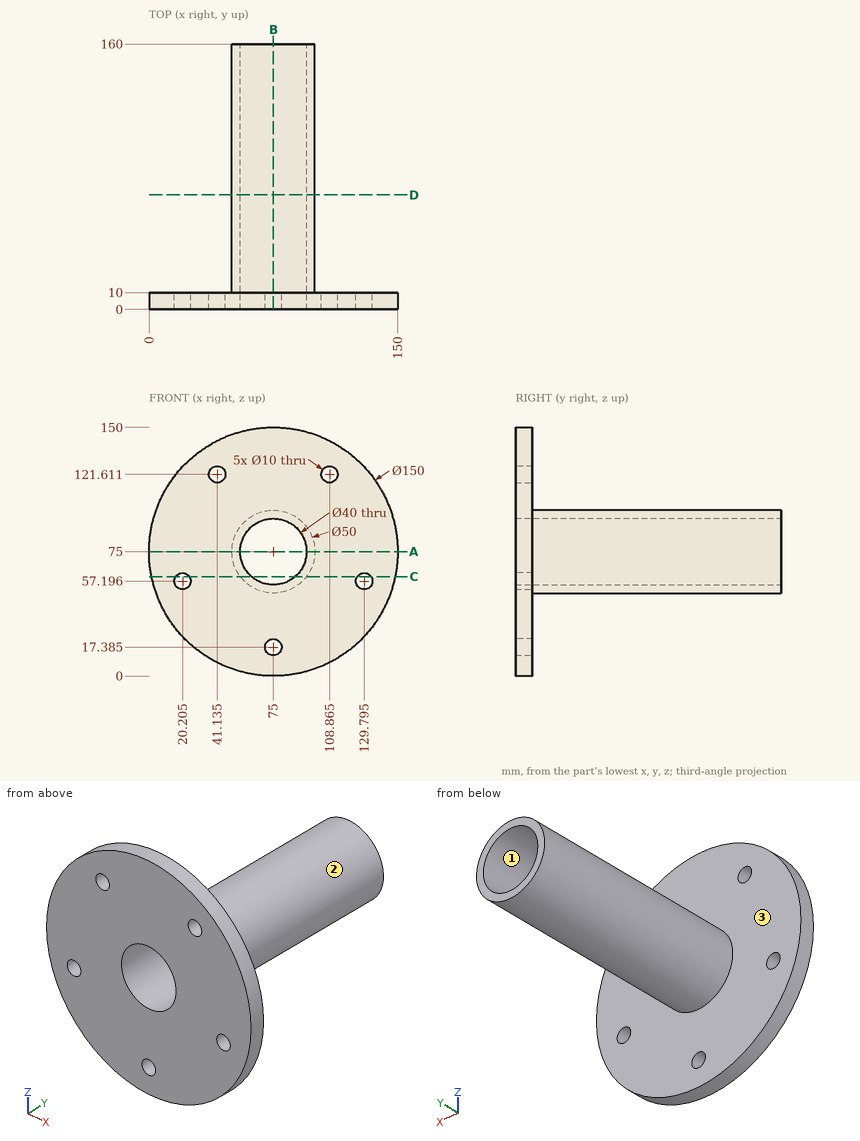
Study the drawing (mm; zero at the part's minimum x, y, z) and answer. Coordinates: 2 decimals unless noted, no trailing zeros. Write each loop counter-clockwise with the first axis right and the second up, starting at its lowest first coordinate (ties: lowest second). Pieces come first, ordered by that corner, then holes.
Q1. A cutting plane is placed at D-D, the plane y = 69. Give the vertices of the cut face in (x, z), then the cut area to 3 significant figures.
Q2. A cutting plane is placed at C-C, the plane z = 60. Give the vertices of the cut face in (x, y) (1 decimal).
Q3. Determine the mould class of the marked faces 1, 2 and 3 for opening direction X: released by +X, released by -X, zero draft, split by the parting line, or undercut.
Q4. A cutting plane is placed at A-A, the plane z = 75. Give the vertices of the cut face in (x, y).
Q5. Each of these flat-tipped pins is pushed along its axis until it touches: pin 1 Ø5 at (y, z) = (33, 96) entering from -X (1 decimal); pin 2 Ø9 at (x, z) = (41.13, 121.61) entering from +Y; pin 3 Ø3 at (y, z) = (100, 94.5) entering from -X; pin 4 Ø4 at (y, z) = (135.5, 97.5) entering from +X. Where does it stop, or does it pass through?
Q6. A cutting plane is placed at B-B, the plane x = 75. Give the vertices of the cut face in (y, z) (1 decimal).
Q7. Find the intervals of material crossed by line 1 (X direction, y = 148, z = 74) (1 decimal); line 2 (Y direction, x = 58, z = 27.5); line 3 (Z direction, x = 60, y = 80.5), in increasing order.
Findings below:
1. outline: circle Ø50 at (75, 75); hole circle Ø40 at (75, 75)
1. area: 707 mm2
2. outline: (1.5, 0) - (16.1, 0) - (16.1, 10) - (1.5, 10) - close; (24.3, 0) - (61.8, 0) - (61.8, 160) - (55, 160) - (55, 10) - (24.3, 10) - close; (88.2, 0) - (125.7, 0) - (125.7, 10) - (95, 10) - (95, 160) - (88.2, 160) - close; (133.9, 0) - (148.5, 0) - (148.5, 10) - (133.9, 10) - close
3. face 1: undercut
3. face 2: split by the parting line
3. face 3: zero draft
4. outline: (0, 0) - (55, 0) - (55, 160) - (50, 160) - (50, 10) - (0, 10) - close; (95, 0) - (150, 0) - (150, 10) - (100, 10) - (100, 160) - (95, 160) - close
5. pin 1: stops at x = 58.2
5. pin 2: passes through
5. pin 3: stops at x = 57.65
5. pin 4: stops at x = 89.31
6. outline: (0, 0) - (10, 0) - (10, 12.4) - (0, 12.4) - close; (0, 22.4) - (10, 22.4) - (10, 50) - (160, 50) - (160, 55) - (0, 55) - close; (0, 95) - (160, 95) - (160, 100) - (10, 100) - (10, 150) - (0, 150) - close
7. line 1: x = 50 to 55, 95 to 100
7. line 2: y = 0 to 10
7. line 3: z = 55 to 61.77, 88.23 to 95
